Read the model definition and answer for the solid it produces. Units are mm, in the model's axes. Face numbers are marked on the shaded views. A direction names the side the tool comes from. Coordinates: 2 decimals unless noted, no trailing zeros. Write each loop counter-clockwise with the first axis right and the second up, starting at its lowest first coordinate (ties: lowest second). Pieces come first, ordered by that corner, then holes.
1) Which of the six approach directions +Z, -Z, +X, -X, +Y, -Y give full straight-line access (tool end or side, diameter ignored) to the marked faces 1, 2 and 3?
2) The part is cut by section A-A (y = -1.25). Determine the outline of the cut face in (x, z).
3) This flat-tipped pin is pushed along its axis until it touches: pin 1 Ø2 at (x, y) = (1, -3) entering from -Z. Where does it stop, or does it pass through?
4) The part is cut by section B-B (x = -13). Determine the outline of the cut face in (y, z).
5) Find the intervals of material crossed by line 1 (X direction, y = 0.5, z = 72), in increasing order.
6) The part is cut by section C-C (z = 76.5). Determine the outline of the cut face in (x, y).
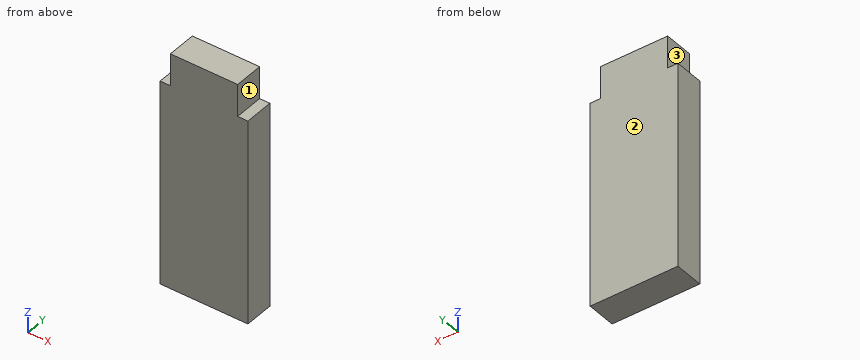
from build123d import *

# Parameters (mm, degrees)
F0_W     = 30
F0_H     = 10
F1_DEPTH = 70
F2_W     = 23
F2_H     = 10
F3_DEPTH = 8
F4_W     = 23
F4_H     = 10
F5_DEPTH = 3


with BuildPart() as f1:
    # F0 (on Top) → F1 (new body)
    with BuildSketch(Plane.XY):
        Rectangle(F0_W, F0_H)
    extrude(amount=F1_DEPTH)

    # F2 (on face) → F3 (join)
    with BuildSketch(Plane.XY.offset(70)):
        Rectangle(F2_W, F2_H)
    extrude(amount=F3_DEPTH)

    # F4 (on face) → F5 (join)
    with BuildSketch(Plane.XY.offset(78)):
        Rectangle(F4_W, F4_H)
    extrude(amount=F5_DEPTH)


solid = f1.part
Reported:
1. face 1: +Z, +X, +Y, -Y
1. face 2: +Z, -Z, +X, -X, +Y
1. face 3: +Z, -X, +Y, -Y
2. outline: (-15, 0) - (15, 0) - (15, 70) - (11.5, 70) - (11.5, 81) - (-11.5, 81) - (-11.5, 70) - (-15, 70) - close
3. pin 1: stops at z = 0
4. outline: (-5, 0) - (5, 0) - (5, 70) - (-5, 70) - close
5. line 1: x = -11.5 to 11.5
6. outline: (-11.5, -5) - (11.5, -5) - (11.5, 5) - (-11.5, 5) - close
